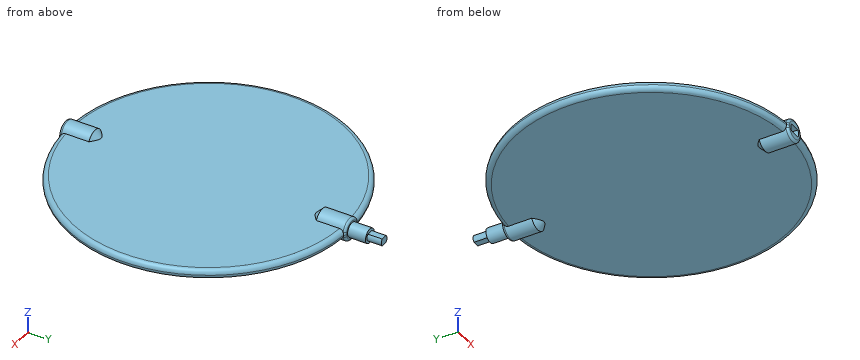
```python
from build123d import *

# Parameters (mm, degrees)
SKETCH018_R     = 59.5
PAD003_DEPTH    = 2
FILLET_R        = 1.999
SKETCH019_R     = 4.6
PAD004_DEPTH    = 15
POCKET007_DEPTH = 10
SKETCH022_R     = 3
PAD005_DEPTH    = 7.5
PAD006_DEPTH    = 6
FILLET001_R     = 1
CHAMFER_SIZE    = 2.599


with BuildPart() as part:
    # Sketch018 (on DatumPlane) → Pad003 (new body, symmetric)
    with BuildSketch(Plane.XY.offset(16.5)):
        Circle(SKETCH018_R)
    extrude(amount=PAD003_DEPTH, both=True)

    # Fillet
    fillet_edges = [part.edges().sort_by_distance(p)[0] for p in [
        (59.5, 0, 16.5),
        (-59.5, 0, 14.5),
        (-59.5, 0, 18.5),
    ]]
    fillet(fillet_edges, radius=FILLET_R)

    # Sketch019 (on DatumPlane) → Pad004 (join)
    with BuildSketch(Plane.XZ.offset(60)):
        with Locations((0, 16.5)):
            Circle(SKETCH019_R)
    pad004 = extrude(amount=-PAD004_DEPTH)

    # Mirrored001: Pad004 across XZ
    add(pad004.mirror(Plane.XZ))

    # Sketch020 (on Face19 of Mirrored001) → Pocket007 (cut)
    with BuildSketch(Plane(origin=(0, -60, 16.5), x_dir=(1, 0, 0), z_dir=(0, -1, 0))):
        with BuildLine():
            Line((-2.210769, 1.55), (2.210769, 1.55))
            ThreePointArc((2.210769, -1.55), (2.7, 0), (2.210769, 1.55))
            Line((-2.210769, -1.55), (2.210769, -1.55))
            ThreePointArc((-2.210769, 1.55), (-2.7, 0), (-2.210769, -1.55))
        make_face()
    extrude(amount=-POCKET007_DEPTH, mode=Mode.SUBTRACT)

    # Sketch022 (on Face8 of Pocket007) → Pad005 (join)
    with BuildSketch(Plane(origin=(0, 60, 16.5), x_dir=(-1, 0, 0), z_dir=(0, 1, 0))):
        Circle(SKETCH022_R)
    extrude(amount=PAD005_DEPTH)

    # Sketch023 (on Face21 of Pad005) → Pad006 (join)
    with BuildSketch(Plane(origin=(0, 67.5, 16.5), x_dir=(-1, 0, 0), z_dir=(0, 1, 0))):
        with BuildLine():
            Line((-1.322876, 1.5), (1.322876, 1.5))
            ThreePointArc((1.322876, -1.5), (2, 0), (1.322876, 1.5))
            Line((-1.322876, -1.5), (1.322876, -1.5))
            ThreePointArc((-1.322876, 1.5), (-2, 0), (-1.322876, -1.5))
        make_face()
    extrude(amount=PAD006_DEPTH)

    # Fillet001
    fillet001_edges = [part.edges().sort_by_distance(p)[0] for p in [
        (-4.6, -60, 16.5),
        (-4.6, 60, 16.5),
    ]]
    fillet(fillet001_edges, radius=FILLET001_R)

    # Chamfer
    chamfer_edges = [part.edges().sort_by_distance(p)[0] for p in [
        (0, 45, 21.1),
        (0, -45, 21.1),
        (0, -45, 11.9),
        (0, 45, 11.9),
    ]]
    chamfer(chamfer_edges, length=CHAMFER_SIZE)


solid = part.part
```
Can you work these out from the model? Positions are in its coordinate system, mm. Give positions to 0.01 mm unless a question says otherwise; leave off trailing zeros. Write each loop counter-clockwise with the first axis right and the second up, starting at its lowest first coordinate (ties: lowest second). Pieces come first, ordered by that corner, then holes. Notation, with made-up numbers: (-35, 81.25) -> (-18, 81.25) arc R23 cw to (-18, 99.25) -> close; hole circle Ø2 at (71, -15). An arc over 180 degrees is marked (long way). One line per item, written item: value.
Q1. Imagine slicing it at A-A on y = 63. Please give me the cut outline in (x, z), and give its area (3 significant figures).
Results found:
outline: circle Ø6 at (0, 16.5)
area: 28.3 mm^2
Q2. For P1, Ø3, axis at x = 0, y = 70.5, coming from the +Z side; P2, Ø1, axis at y = -31, z = 18.5, coming from the -X side; P3, Ø0.8, axis at x = 0.5, y = 69.5, coming from the -Z side, each with a flat end and sliding along its axis, tell me the tip position at first contact or that it passes through.
Results found:
P1: stops at z = 18
P2: stops at x = -50.06
P3: stops at z = 15
Q3. Please list where these lines run through material, in increasing order: line 1 (Z direction, x = 51.5, y = -23); line 2 (Y direction, x = -7, z = 16); line 3 (X direction, y = 61.5, z = 18.75). Write a range as [from, to].
Results found:
line 1: z = [14.5, 18.5]
line 2: y = [-59.02, 59.02]
line 3: x = [-1.98, 1.98]
